For this review, take the finished solid that the model builds, in its own axes (mm). Face numbers are marked on the shaded views. A direction names the side the tool comes from. Round coordinates to 2 decimals unless told otherwise and drop trailing zeros. Write each loop counter-clockwise with the first axis right and the second up, starting at its lowest first coordinate (ties: lowest second). Pieces come first, ordered by that corner, then holes. Notation, with made-up numbers: M 86.25,-38.5 L 121.25,-38.5 A20 cw 121.25,-31.5 Z; hole C 29,-15.5 d8. An arc over 180 degrees is marked long. Use one line per item in the form item = value. Start each with the question number.
Item 1: For line 1 (Z direction, x = 0.9, y = -2.15); line 2 (Y direction, x = 0, z = 4.35); line 3 (X direction, y = -0.8, z = 4.7), list the stretches that pass through material, from the lowest coordinate up. Write a range as [from, to].
Item 2: Add section A-A (z = 2.85). State the section outline as (x, y) points, and give its area (3 significant figures).
Item 3: Add section C-C (x = 0). State the section outline as (y, z) points, and give its area (3 significant figures).
Item 4: Add section D-D (x = 1.6). State the section outline as (y, z) points, and give its area (3 significant figures).
Item 5: Draft analysis for pull direction Z (two halves, no side actions). For the marked faces 5, 6, 7 and 8, state which applies: released by +Z, released by -Z, zero draft, split by the parting line, or undercut.
Item 6: For P1, Ø1.5, axis at x = -0.5, y = 0, coming from the -Z side; P2, Ø3, axis at x = -1.5, z = 3.5, coming from the -Y side; P3, Ø1.2, axis at x = 0, y = 0, coming from the +Z side, all flat-tipped, find the tip position at first contact; note any pin that passes through.
Item 7: Add section B-B (y = 0.8). State the section outline as (x, z) points, and give its area (3 significant figures).
Item 8: For the marked faces 1, 2, 3 and 4, list the 3-axis set-ups (+Z, -Z, +X, -X, +Y, -Y) from which the entire face can be reached by the end or side of a thin tool; tool diameter is ignored.
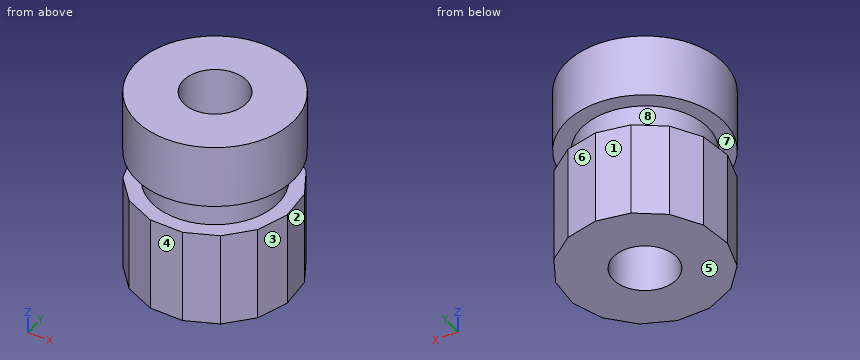
Autodesk Inventor part; units mm, degrees
ref_plane "YZ Plane" through (0, 0, 0) normal (1, 0, 0) x (0, 1, 0)
ref_plane "XZ Plane" through (0, 0, 0) normal (0, 1, 0) x (-1, 0, 0)
ref_plane "XY Plane" through (0, 0, 0) normal (0, 0, 1) x (1, 0, 0)
sketch "Sketch1" plane through (0, 0, 0) normal (0, 0, 1) x (1, 0, 0)
  line L0 (2.4094, 0.6671) -> (2.4724, -0.3706)
  line L1 (2.4724, -0.3706) -> (2.1079, -1.3442)
  line L2 (2.1079, -1.3442) -> (1.3789, -2.0853)
  line L3 (1.3789, -2.0853) -> (0.4116, -2.4659)
  line L4 (0.4116, -2.4659) -> (-0.627, -2.4201)
  line L5 (-0.627, -2.4201) -> (-1.5571, -1.9558)
  line L6 (-1.5571, -1.9558) -> (-2.218, -1.1534)
  line L7 (-2.218, -1.1534) -> (-2.4954, -0.1515)
  line L8 (-2.4954, -0.1515) -> (-2.3413, 0.8765)
  line L9 (-2.3413, 0.8765) -> (-1.7824, 1.753)
  line L10 (-1.7824, 1.753) -> (-0.9153, 2.3264)
  line L11 (-0.9153, 2.3264) -> (0.1101, 2.4976)
  line L12 (0.1101, 2.4976) -> (1.1165, 2.2369)
  line L13 (1.1165, 2.2369) -> (1.9297, 1.5894)
  line L14 (1.9297, 1.5894) -> (2.4094, 0.6671)
  circle A0 centre (0, 0) radius 1
  dimension "d1" = 2
extrude "Extrusion1" add sketch "Sketch1" along normal blind 3
sketch "Sketch2" plane through (0, 0, 3) normal (0, 0, 1) x (1, 0, 0)
  circle A0 centre (0, 0) radius 1
  line L0 (2.4724, -0.3706) -> (2.4094, 0.6671)
  line L1 (2.4094, 0.6671) -> (1.9297, 1.5894)
  line L2 (1.9297, 1.5894) -> (1.1165, 2.2369)
  line L3 (1.1165, 2.2369) -> (0.1101, 2.4976)
  line L4 (0.1101, 2.4976) -> (-0.9153, 2.3264)
  line L5 (-0.9153, 2.3264) -> (-1.7824, 1.753)
  line L6 (-1.7824, 1.753) -> (-2.3413, 0.8765)
  line L7 (-2.3413, 0.8765) -> (-2.4954, -0.1515)
  line L8 (-2.4954, -0.1515) -> (-2.218, -1.1534)
  line L9 (-2.218, -1.1534) -> (-1.5571, -1.9558)
  line L10 (-1.5571, -1.9558) -> (-0.627, -2.4201)
  line L11 (-0.627, -2.4201) -> (0.4116, -2.4659)
  line L12 (0.4116, -2.4659) -> (1.3789, -2.0853)
  line L13 (1.3789, -2.0853) -> (2.1079, -1.3442)
  line L14 (2.1079, -1.3442) -> (2.4724, -0.3706)
  circle A1 centre (0, 0) radius 2
  dimension "d4" = 4
extrude "Extrusion2" add sketch "Sketch2" along normal blind 1 contours A1
sketch "Sketch3" plane through (0, 0, 4) normal (0, 0, 1) x (1, 0, 0)
  circle A0 centre (0, 0) radius 1
  circle A1 centre (0, 0) radius 2
  circle A2 centre (0, 0) radius 2.5
  dimension "d7" = 5
extrude "Extrusion3" add sketch "Sketch3" along normal blind 2 contours A1 | A2
properties part number "servo 2"
Calculated:
q1.line_1 = [0, 3], [4, 6]
q1.line_2 = [-2.5, -1], [1, 2.5]
q1.line_3 = [-2.37, -0.6], [0.6, 2.37]
q2.outline = M -2.5,-0.15 L -2.22,-1.15 L -1.56,-1.96 L -0.63,-2.42 L 0.41,-2.47 L 1.38,-2.09 L 2.11,-1.34 L 2.47,-0.37 L 2.41,0.67 L 1.93,1.59 L 1.12,2.24 L 0.11,2.5 L -0.92,2.33 L -1.78,1.75 L -2.34,0.88 Z; hole C 0,0 d2
q2.area = 15.9 mm^2
q3.outline = M -2.5,4 L -2,4 L -2,3 L -2.45,3 L -2.45,0 L -1,0 L -1,6 L -2.5,6 Z; M 1,0 L 2.48,0 L 2.48,3 L 2,3 L 2,4 L 2.5,4 L 2.5,6 L 1,6 Z
q3.area = 16.8 mm^2
q4.outline = M -1.92,4 L -1.2,4 L -1.2,3 L -1.86,3 L -1.86,0 L 1.85,0 L 1.85,3 L 1.2,3 L 1.2,4 L 1.92,4 L 1.92,6 L -1.92,6 Z
q4.area = 21.2 mm^2
q5.face_5 = released by -Z
q5.face_6 = zero draft
q5.face_7 = undercut
q5.face_8 = undercut
q6.P1 = 0
q6.P2 = -2.5
q6.P3 = through
q7.outline = M -2.37,4 L -1.83,4 L -1.83,3 L -2.35,3 L -2.35,0 L -0.6,0 L -0.6,6 L -2.37,6 Z; M 0.6,0 L 2.34,0 L 2.34,3 L 1.83,3 L 1.83,4 L 2.37,4 L 2.37,6 L 0.6,6 Z
q7.area = 20.0 mm^2
q8.face_1 = -Z, -X, +Y
q8.face_2 = -Z, +X, +Y
q8.face_3 = -Z, +X, -Y
q8.face_4 = -Z, -X, -Y
